```python
from build123d import *

# Parameters (mm, degrees)
SKETCH_8_R          = 1.05
EXTRUDE_4_DEPTH     = 1.5
SKETCH_14_W         = 2.317821063
SKETCH_14_H         = 10.810249676
CUT_EXTRUDE_3_DEPTH = 4
CUT_EXTRUDE_5_DEPTH = 4
FILLET_3_R          = 1


with BuildPart() as part:
    # 草图8 → 凸台-拉伸4 (new body, symmetric)
    with BuildSketch(Plane(origin=(0, 0, 0), x_dir=(0, 0, -1), z_dir=(1, 0, 0))):
        with BuildLine():
            Line((1.5, 2.598076211), (-10.624355653, 9.598076211))
            ThreePointArc((-10.624355653, 9.598076211), (-13.829953141, 3.705724776), (-14, -3))
            Line((-14, -3), (0, -3))
            ThreePointArc((0, -3), (2.897777479, -0.776457135), (1.5, 2.598076211))
        make_face()
        Circle(SKETCH_8_R, mode=Mode.SUBTRACT)
    extrude(amount=EXTRUDE_4_DEPTH, both=True)

    # 草图14 → 切除-拉伸3 (cut, through all)
    with BuildSketch(Plane(origin=(1.5, 0, 0), x_dir=(0, 0, -1), z_dir=(1, 0, 0))):
        with Locations((-13.158910532, 2.405124838)):
            Rectangle(SKETCH_14_W, SKETCH_14_H)
    extrude(amount=-CUT_EXTRUDE_3_DEPTH, mode=Mode.SUBTRACT)

    # 草图17 → 切除-拉伸5 (cut, through all)
    with BuildSketch(Plane(origin=(1.5, 0, 0), x_dir=(0, 0, -1), z_dir=(1, 0, 0))):
        with BuildLine():
            ThreePointArc((-7.014805771, 4.05), (-7.823999193, 2.096434265), (-8.1, 0))
            ThreePointArc((-8.1, 0), (-7, -1.1), (-5.9, 0))
            ThreePointArc((-5.9, 0), (-5.698962375, 1.527032366), (-5.109549882, 2.95))
            ThreePointArc((-5.109549882, 2.95), (-5.512177826, 4.452627944), (-7.014805771, 4.05))
        make_face()
    extrude(amount=-CUT_EXTRUDE_5_DEPTH, mode=Mode.SUBTRACT)

    # 圆角3
    fillet_3_edges = [part.edges().sort_by_distance(p)[0] for p in [
        (0, -3, 12),
        (0, 7.810249676, 12),
        (0, 9.598076211, 10.624355653),
    ]]
    fillet(fillet_3_edges, radius=FILLET_3_R)


solid = part.part
```
For this review, take the finished solid that the model builds, in its own axes (mm). A direction names the side the tool comes from. Coordinates: 2 decimals unless noted, no trailing zeros. Loops run counter-clockwise (first coordinate to the right, second up) from the corner with the lowest first, then second, coordinate; pieces in that order, holes last. Notation, with made-up numbers: (84.5, -30.5) - (101.5, -30.5) arc R10 ccw to (101.5, -26.5) - close; hole circle Ø7 at (-38.75, 43.25). An arc over 180 degrees is marked (long way). Use one line per item in the form item = value. Start each with the question number.
1) For faces 1 (the face through (-0.021, -2.715, 11.699)), 2 (the face through (0.021, 2.125, 7.816)), list the 3-axis set-ups (+Z, -Z, +X, -X, +Y, -Y) from which the entire face can be reached by the end or side of a thin tool; tool diameter is ignored.
2) To check wall thickness, follow probe 1 along Y at (x, z) = (-0.05, 0); probe 2 along Z at (x, y) = (-1.05, 2); probe 3 along Z at (x, y) = (-0.2, 3.75). State the ranges of each line that lie inside material, in increasing order. Write a range as from..to.
3) Take a section at A-A (x = 0.3). State the section outline as (y, z) points.
4) Take a section at B-B (y = 3.5). State the section outline as (x, z) points, plus the area to 3 significant figures.
5) Take a section at D-D (y = 5.5). State the section outline as (x, z) points, plus the area to 3 significant figures.
6) For pin 1 (4 mm diameter, centred on y = 3.5, z = 6, fed in from +X), flat-tipped, find the tip position at first contact; note if it passes through.
7) Take a section at C-C (z = 0.5). State the section outline as (x, y) points.
8) Draft analysis for pull direction Y (two halves, no side actions). For faces 3 (the face through (0, -1.1, 7)), 4 (the face through (0.021, 8.518, 11.509)), 5 (the face through (1.5, 2, 5)), state which applies: released by +Y, released by -Y, zero draft, split by the parting line, or undercut.
From the geometry:
q1.face_1 = +Z, +X, -X, -Y
q1.face_2 = +X, -X
q2.probe_1 = -3..-1.05, 1.05..3.46
q2.probe_2 = -2.24..5.55, 7.85..12
q2.probe_3 = 0.5..4.99, 7.18..12
q3.outline = (-3, 0) arc R3 ccw to (2.6, -1.5) - (9.18, 9.9) arc R1 ccw to (8.94, 11.18) arc R14.32 ccw to (8.07, 11.83) arc R1 ccw to (7.51, 12) - (-2, 12) arc R1 ccw to (-3, 11) - close; hole circle Ø2.1 at (0, 0); hole (0, 5.9) arc R5.9 cw to (2.95, 5.11) arc R1.1 ccw to (4.05, 7.01) arc R8.1 ccw to (0, 8.1) arc R1.1 ccw to start
q4.outline = (-1.5, 0.06) - (1.5, 0.06) - (1.5, 4.96) - (-1.5, 4.96) - close; (-1.5, 7.3) - (1.5, 7.3) - (1.5, 12) - (-1.5, 12) - close
q4.area = 28.8 mm2
q5.outline = (-1.5, 3.53) - (1.5, 3.53) - (1.5, 12) - (-1.5, 12) - close
q5.area = 25.4 mm2
q6.pin_1 = 1.5
q7.outline = (-1.5, -3) - (1.5, -3) - (1.5, -0.92) - (-1.5, -0.92) - close; (-1.5, 0.92) - (1.5, 0.92) - (1.5, 3.75) - (-1.5, 3.75) - close
q8.face_3 = undercut
q8.face_4 = released by +Y
q8.face_5 = zero draft
